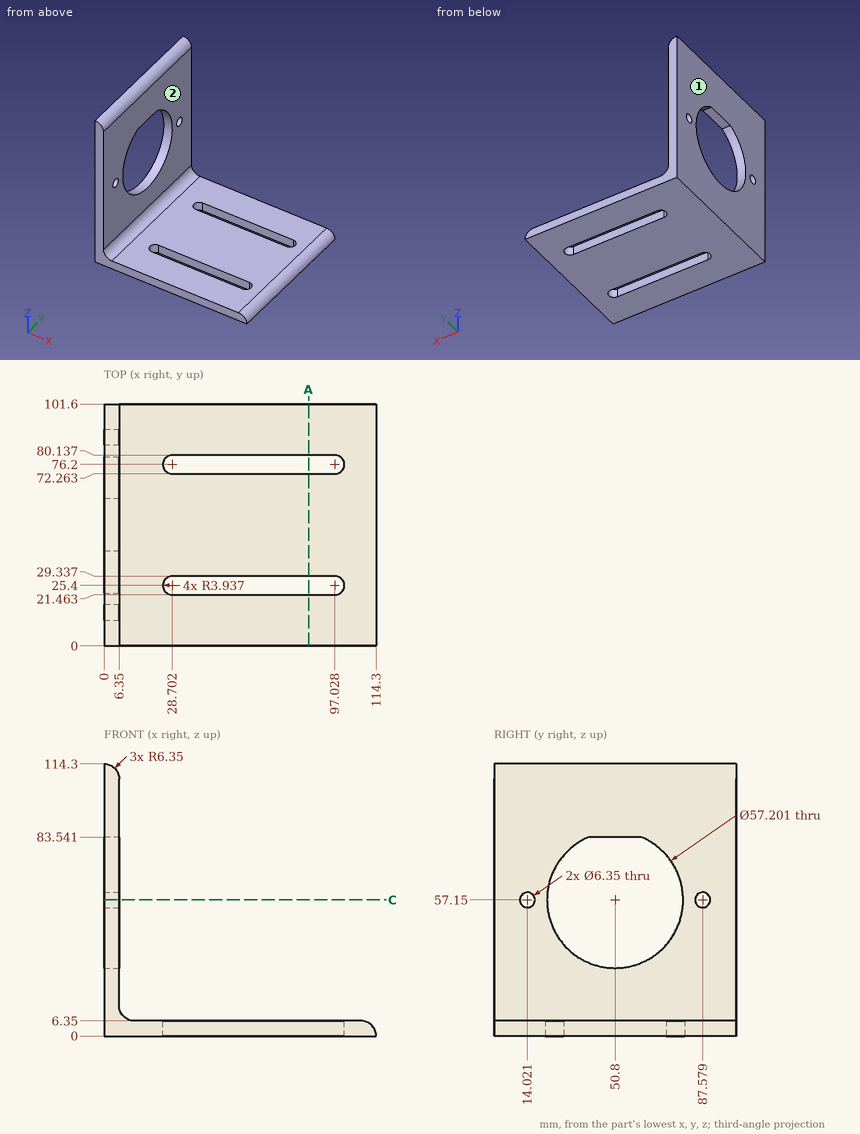
Study the drawing (mm; zero at the part's minimum x, y, z) and answer. A direction names the side the tool comes from. Coordinates: 2 decimals unless noted, no trailing zeros. Write each loop counter-clockwise with the first axis right and the second up, starting at its lowest first coordinate (ties: lowest second). Pieces come first, ordered by that corner, then holes. Notation, with made-up numbers: M 45,80.25 L 61,80.25 A29 ccw 61,114.25 Z; hole C 18,-1.75 d3. An arc over 180 degrees is marked long. Use a Markdown table: item, result. Add a question column.
1. Straight lines are drawn through the part: line 1 along Y through (x, z) = (4, 57); line 2 along X through (y, z) = (35, 82). For each, find the intervals that lie inside material, in ascending order. Write a range as [from, to].
2. Which of the six approach directions +Z, -Z, +X, -X, +Y, -Y give full straight-line access (tool end or side, diameter ignored) to the marked faces 1 and 2?
3. Section C-C (z = 57.15) is taken. Count the separate pieces of the cut face and the enclosed holes in it, plus the area to 3 significant figures.
4. Section A-A (x = 86) is taken. Give the vertices of the cut face in (y, z), plus the area to 3 significant figures.
5. Given P1, Ø8.5, axis at y = 87.58, z = 57.15, coming from the +X side; P2, Ø10, axis at x = 75, y = 40.5, coming from the +Z side; P3, Ø5.5, axis at y = 14.02, z = 57.15, coming from the -X side, each flat-ended and moving along its own axis, determine where each tip first touches the part or whether it passes through.
Data:
| question | item | result |
|---|---|---|
| 1 | line 1 | y = [0, 10.85], [17.19, 22.2], [79.4, 84.41], [90.75, 101.6] |
| 1 | line 2 | x = [0, 6.35] |
| 2 | face 1 | +Z, -Z, -X, +Y, -Y |
| 2 | face 2 | +Z, +X, +Y, -Y |
| 3 | separate pieces | 4 |
| 3 | enclosed holes | 0 |
| 3 | area | 201 mm2 |
| 4 | outline | M 0,0 L 21.46,0 L 21.46,6.35 L 0,6.35 Z; M 29.34,0 L 72.26,0 L 72.26,6.35 L 29.34,6.35 Z; M 80.14,0 L 101.6,0 L 101.6,6.35 L 80.14,6.35 Z |
| 4 | area | 545 mm2 |
| 5 | P1 | stops at x = 6.35 |
| 5 | P2 | stops at z = 6.35 |
| 5 | P3 | passes through |
